```python
from build123d import *

# Parameters (mm, degrees)
SKETCH1_W           = 80
SKETCH1_H           = 3
BOSS_EXTRUDE1_DEPTH = 30


with BuildPart() as part:
    # Sketch1 → Boss-Extrude1 (new body)
    with BuildSketch(Plane.XY):
        with BuildLine():
            Line((74, 3), (80, 3))
            Line((80, 3), (80, 63))
            ThreePointArc((80, 63), (77, 60), (74, 63))
            Line((74, 63), (74, 3))
        make_face()
        with BuildLine():
            Line((78.75, 63), (80, 63))
            ThreePointArc((80, 63), (79.557579886, 64.568051379), (78.360809916, 65.673611111))
            Line((78.360809916, 65.673611111), (75.639190084, 65.673611111))
            ThreePointArc((75.639190084, 65.673611111), (74.442420114, 64.568051379), (74, 63))
            Line((74, 63), (75.25, 63))
            ThreePointArc((75.25, 63), (77, 64.75), (78.75, 63))
        make_face()
        with BuildLine():
            ThreePointArc((74, 63), (77, 60), (80, 63))
            Line((80, 63), (78.75, 63))
            ThreePointArc((78.75, 63), (77, 61.25), (75.25, 63))
            Line((75.25, 63), (74, 63))
        make_face()
        with BuildLine():
            Line((75.639190084, 65.673611111), (78.360809916, 65.673611111))
            ThreePointArc((78.360809916, 65.673611111), (77, 66), (75.639190084, 65.673611111))
        make_face()
        with BuildLine():
            ThreePointArc((6, 9), (3, 12), (0, 9))
            Line((0, 9), (1.25, 9))
            ThreePointArc((1.25, 9), (3, 10.75), (4.75, 9))
            Line((4.75, 9), (6, 9))
        make_face()
        with BuildLine():
            Line((1.25, 9), (0, 9))
            ThreePointArc((0, 9), (3, 6), (6, 9))
            Line((6, 9), (4.75, 9))
            ThreePointArc((4.75, 9), (3, 7.25), (1.25, 9))
        make_face()
        with BuildLine():
            Line((0, 9), (0, 3))
            Line((0, 3), (6, 3))
            Line((6, 3), (6, 9))
            ThreePointArc((6, 9), (3, 6), (0, 9))
        make_face()
        with Locations((40, 1.5)):
            Rectangle(SKETCH1_W, SKETCH1_H)
    extrude(amount=BOSS_EXTRUDE1_DEPTH)


solid = part.part
```
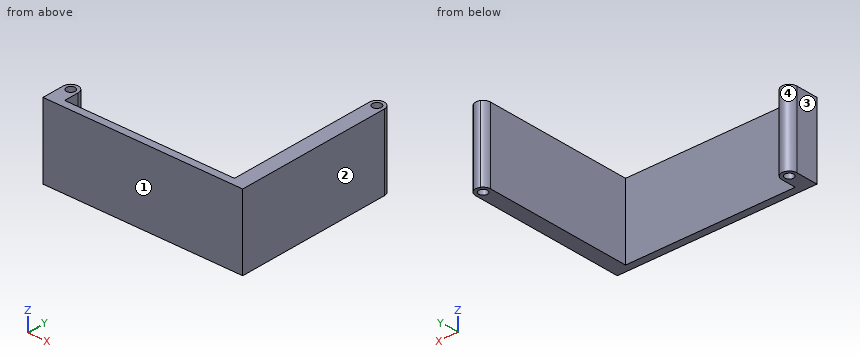
Can you work these out from the model? Positions are in its coordinate system, mm. Face numbers are marked on the shaded views. Coordinates: 2 decimals unless noted, no trailing zeros. Write each loop counter-clockwise with the first axis right and the second up, starting at its lowest first coordinate (ties: lowest second). Pieces come first, ordered by that corner, then holes. Notation, with made-up numbers: M -37,55 L -7,55 A24 ccw -7,77 Z; hole C 24,-0.5 d10. An arc over 180 degrees is marked long. Write item = value, one per line. Start each with the question number.
Q1. I'm going to push flat-ended pins straight in: pin 1 (1 mm diameter, centred on x = 52.5, z = 4, fed in from +Y); pin 2 (1 mm diameter, centred on y = 51, z = 5, fed in from -X); pin 3 (3 mm diameter, centred on x = 3, y = 9, fed in from +Z). Where does each tip first touch, or does it pass through?
Q2. If I drill on L1, parallel to X at y = 9, z = 6; L2, parallel to Y at x = 3, z = 17.5; L3, parallel to Y at x = 77, z = 14.75, over which ranges is the centre line in solid material (lowest first)? Write a range as [from, to].
Q3. Thinking about a two-plate mould opening in X: for the marked faces 1, 2, 3 and 4, which applies, released by +X, released by -X, zero draft, split by the parting line, or undercut?
Q4. If we section it at B-B, the plane z = 7: Write out the boundary of the cut face in (x, y).
Q5. If we section it at D-D, the plane x = 69: Write out the boundary of the cut face in (y, z), then the cut area to 3 significant figures.
Q6. If we section it at A-A, the plane x = 3: Write out the boundary of the cut face in (y, z), then the cut area to 3 significant figures.
Q7. If we section it at C-C, the plane x = 77: Write out the boundary of the cut face in (y, z), then the cut area to 4 significant figures.
Check sheet entries:
q1.pin_1 = 3
q1.pin_2 = 74
q1.pin_3 = through
q2.L1 = [0, 1.25], [4.75, 6], [74, 80]
q2.L2 = [0, 7.25], [10.75, 12]
q2.L3 = [0, 61.25], [64.75, 66]
q3.face_1 = zero draft
q3.face_2 = released by +X
q3.face_3 = released by -X
q3.face_4 = undercut
q4.outline = M 0,0 L 80,0 L 80,63 A3 ccw 74,63 L 74,3 L 6,3 L 6,9 A3 ccw 0,9 Z; hole C 3,9 d3.5; hole C 77,63 d3.5
q5.outline = M 0,0 L 3,0 L 3,30 L 0,30 Z
q5.area = 90.0 mm²
q6.outline = M 0,0 L 7.25,0 L 7.25,30 L 0,30 Z; M 10.75,0 L 12,0 L 12,30 L 10.75,30 Z
q6.area = 255 mm²
q7.outline = M 0,0 L 61.25,0 L 61.25,30 L 0,30 Z; M 64.75,0 L 66,0 L 66,30 L 64.75,30 Z
q7.area = 1,875 mm²
